Check sheet for the drawn part. Datum: minimum x, y, z corner. Units: mm. Coordinates: 2 decimals unless noted, no trailing zeros. Write each loop counter-clockwise with the first axis right and the second up, starting at its lowest first coordinate (ties: lowest second). Pieces come first, ordered by that corner, then holes. Notation, with made-up numbers: (24, -20) -> (28, -20) arc R24 ccw to (28, 16) -> close; hole circle Ø8 at (-34, 73). An arc over 180 degrees is marked (long way). Answer in a Markdown table with one row per item. Add a question column.
Q1. Thickness scan on line 1 (Z direction, x = 72.5, y = 2.25); line 2 (X direction, y = 5.5, z = 67.5); line 3 (Z direction, x = 14, y = 3.5). Record the ranges inside material, lowest first.
Q2. Section check A-A, the plane y = 4.75. Record the boundary of the cut face in (x, z).
Q3. Section check B-B, the plane x = 6. Record the boundary of the cut face in (y, z).
Q4. Gauge pin test, flat end, axial feed: P1, Ø1.5, axis at x = 73, y = 3.5, coming from the +Z side. Record the tip position at first contact, or that the pin passes through.
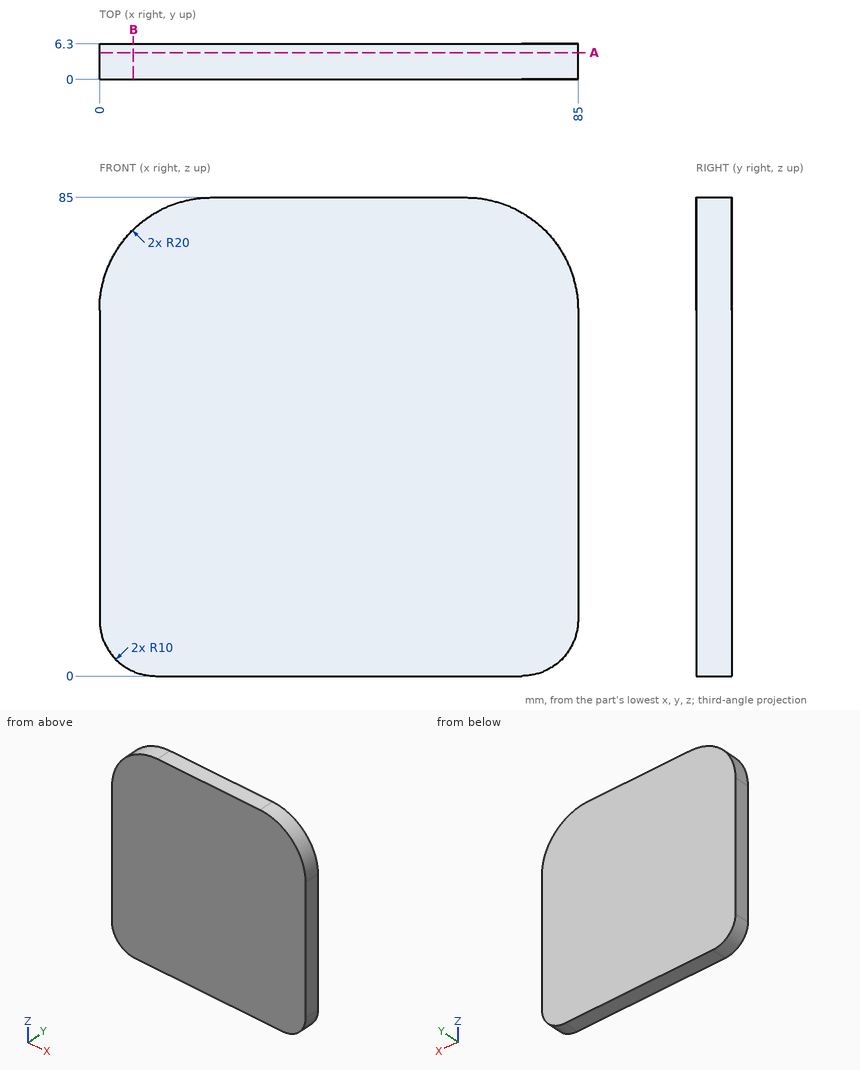
Calculated:
| question | item | result |
|---|---|---|
| 1 | line 1 | z = 0 to 83.54 |
| 1 | line 2 | x = 0.16 to 84.84 |
| 1 | line 3 | z = 0 to 84.08 |
| 2 | outline | (0, 10) arc R10 ccw to (10, 0) -> (75, 0) arc R10 ccw to (85, 10) -> (85, 65) arc R20 ccw to (65, 85) -> (20, 85) arc R20 ccw to (0, 65) -> close |
| 3 | outline | (0, 0.83) -> (6.3, 0.83) -> (6.3, 79.28) -> (0, 79.28) -> close |
| 4 | P1 | stops at z = 83.64 |
